Verification items for the finished model (mm, model axes). Give positions to 0.01 mm unless a question says otherwise; leave off trailing zeros. Order: outer loops, then holes, each group sorted by start corner. A loop starts at its lowest first (then second) coordinate and runs counter-clockwise, first axis right, second up.
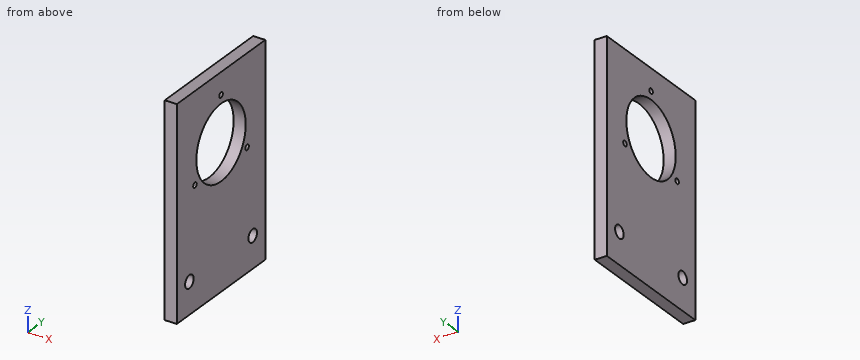
from build123d import *

# Parameters (mm, degrees)
SKETCH1_W           = 69.85
SKETCH1_H           = 110
SKETCH1_R           = 19.5
SKETCH1_R_2         = 3.37312
SKETCH1_R_3         = 1.4
BOSS_EXTRUDE1_DEPTH = 6.35


with BuildPart() as part:
    # Sketch1 → Boss-Extrude1 (new body)
    with BuildSketch(Plane.YZ):
        Rectangle(SKETCH1_W, SKETCH1_H)
        with Locations((0, 19.75)):
            Circle(SKETCH1_R, mode=Mode.SUBTRACT)
        with Locations((-25, -38.4)):
            Circle(SKETCH1_R_2, mode=Mode.SUBTRACT)
        with Locations((25, -38.4)):
            Circle(SKETCH1_R_2, mode=Mode.SUBTRACT)
        with Locations((0, 43.5)):
            Circle(SKETCH1_R_3, mode=Mode.SUBTRACT)
        with Locations((20.56810334, 7.875)):
            Circle(SKETCH1_R_3, mode=Mode.SUBTRACT)
        with Locations((-20.56810334, 7.875)):
            Circle(SKETCH1_R_3, mode=Mode.SUBTRACT)
    extrude(amount=BOSS_EXTRUDE1_DEPTH)


solid = part.part
(1) Scan lines: line 1 (Z direction, x = 3.5, y = -25); line 2 (Y direction, x = 3.75, z = 19.5) (3 decimals); line 3 (Z direction, x = 2.5, y = -1). Record each from-to range of solid material in increasing order.
Solved:
line 1: z = -55 to -41.77, -35.03 to 55
line 2: y = -34.925 to -19.498, 19.498 to 34.925
line 3: z = -55 to 0.28, 39.22 to 42.52, 44.48 to 55
(2) Section check B-B, the plane y = -25. Enter the section's corners in (x, z).
Solved:
outline: (0, -55) - (6.35, -55) - (6.35, -41.77) - (0, -41.77) - close; (0, -35.03) - (6.35, -35.03) - (6.35, 55) - (0, 55) - close
(3) Section check D-D, the plane y = 0. Enter the section's corners in (x, z), then the cut area to 3 significant figures.
Solved:
outline: (0, -55) - (6.35, -55) - (6.35, 0.25) - (0, 0.25) - close; (0, 39.25) - (6.35, 39.25) - (6.35, 42.1) - (0, 42.1) - close; (0, 44.9) - (6.35, 44.9) - (6.35, 55) - (0, 55) - close
area: 433 mm2
(4) Section check A-A, the plane z = -38.4. Enter the section's corners in (x, y) (3 decimals), then the cut area to 3 significant figures.
Solved:
outline: (0, -34.925) - (6.35, -34.925) - (6.35, -28.373) - (0, -28.373) - close; (0, -21.627) - (6.35, -21.627) - (6.35, 21.627) - (0, 21.627) - close; (0, 28.373) - (6.35, 28.373) - (6.35, 34.925) - (0, 34.925) - close
area: 358 mm2
(5) Section check C-C, the plane z = 19.75. Enter the section's corners in (x, y) (3 decimals).
Solved:
outline: (0, -34.925) - (6.35, -34.925) - (6.35, -19.5) - (0, -19.5) - close; (0, 19.5) - (6.35, 19.5) - (6.35, 34.925) - (0, 34.925) - close
